from build123d import *

# Parameters (mm, degrees)
SKETCH1_R                = 11.1125
BOSS_EXTRUDE1_DEPTH      = 38.1
BOSS_EXTRUDE2_DEPTH      = 12.7
BOSS_EXTRUDE2_DEPTH_BACK = 12.7
SKETCH2_W                = 9.525
SKETCH2_H                = 31.75
BOSS_EXTRUDE3_DEPTH      = 12.7
BOSS_EXTRUDE3_DEPTH_BACK = 12.7
SKETCH3_W                = 63.5
SKETCH3_H                = 12.7
BOSS_EXTRUDE4_DEPTH      = 12.7
BOSS_EXTRUDE4_DEPTH_BACK = 12.7
SKETCH4_W                = 9.525
SKETCH4_H                = 63.5
BOSS_EXTRUDE5_DEPTH      = 12.7
BOSS_EXTRUDE5_DEPTH_BACK = 12.7


with BuildPart() as part:
    # Sketch1 → Boss-Extrude1 (new body)
    with BuildSketch(Plane(origin=(0, 0, 0), x_dir=(0, 0, -1), z_dir=(1, 0, 0))):
        Circle(SKETCH1_R)
    extrude(amount=-BOSS_EXTRUDE1_DEPTH)

    # Sketch2 → Boss-Extrude2 (add, two sides: drawn at the far end of the back side and taken through both)
    with BuildSketch(Plane.XY.offset(-BOSS_EXTRUDE2_DEPTH_BACK)):
        with Locations((4.7625, 4.7625)):
            Rectangle(SKETCH2_W, SKETCH2_H)
    extrude(amount=BOSS_EXTRUDE2_DEPTH + BOSS_EXTRUDE2_DEPTH_BACK)

    # Sketch3 → Boss-Extrude3 (add, two sides: drawn at the far end of the back side and taken through both)
    with BuildSketch(Plane.XY.offset(-BOSS_EXTRUDE3_DEPTH_BACK)):
        with Locations((-22.225, 26.9875)):
            Rectangle(SKETCH3_W, SKETCH3_H)
    extrude(amount=BOSS_EXTRUDE3_DEPTH + BOSS_EXTRUDE3_DEPTH_BACK)

    # Sketch4 → Boss-Extrude4 (add, two sides: drawn at the far end of the back side and taken through both)
    with BuildSketch(Plane.XY.offset(-BOSS_EXTRUDE4_DEPTH_BACK)):
        with Locations((-49.2125, 52.3875)):
            Rectangle(SKETCH4_W, SKETCH4_H)
    extrude(amount=BOSS_EXTRUDE4_DEPTH + BOSS_EXTRUDE4_DEPTH_BACK)

    # Sketch5 → Boss-Extrude5 (add, two sides: drawn at the far end of the back side and taken through both)
    with BuildSketch(Plane.XY.offset(-BOSS_EXTRUDE5_DEPTH_BACK)):
        Polygon((-53.975, 71.4375), (-41.23944, 71.4375), (-41.23944, 74.6125), (-28.575, 74.6125), (-28.575, 84.1375), (-53.975, 84.1375), align=None)
    extrude(amount=BOSS_EXTRUDE5_DEPTH + BOSS_EXTRUDE5_DEPTH_BACK)


solid = part.part
Design review of the part built by this model. Coordinates are the model's own, in mm. A direction names the side the tool comes from. Coordinates: 2 decimals unless noted, no trailing zeros. Loops run counter-clockwise (first coordinate to the right, second up) from the corner with the lowest first, then second, coordinate; pieces in that order, holes last. Notation, with made-up numbers: M 51,-17.75 L 73,-17.75 A27 cw 73,13.25 Z; hole C 85.5,21 d4. An arc over 180 degrees is marked long. Use one line per item in the form item = value.
(1) Consider section B-B (x = -11). Write out the cut boundary in (y, z) (1 decimal).
Return value:
outline = C 0,0 d22.2; M 20.6,-12.7 L 33.3,-12.7 L 33.3,12.7 L 20.6,12.7 Z
(2) For line 1 along Y through (x, z) = (-32.5, 4); line 2 along Y through (x, z) = (4.5, 2.75); line 3 along Y through (x, z) = (-19.5, 2.25), list the stretches that pass through material, from the lowest coordinate up. Write a range as from..to.
Return value:
line_1 = -10.37..10.37, 20.64..33.34, 74.61..84.14
line_2 = -11.11..33.34
line_3 = -10.88..10.88, 20.64..33.34
(3) Draft analysis for pull direction Y (two halves, no side actions). For faces 1 (the face through (9.525, 11, 0)), 2 (the face through (-41, 84.138, 0)), 3 (the face through (-27, 20.638, 0)), 4 (the face through (5, -11.112, 0)), state which applies: pulls with the +Y half, pulls with the -Y half, needs draft (parallel to the pull), parting line crosses it, or undercut.
Return value:
face_1 = needs draft
face_2 = pulls with the +Y half
face_3 = undercut
face_4 = pulls with the -Y half
(4) Clearance check with flat-ended pins moving along their axes: P1, Ø1.6, axis at y = 73.5, z = 2, coming from the +X side; P2, Ø2.5, axis at x = -42.5, z = -5.5, coming from the -Y side; P3, Ø10, axis at y = 33.5, z = -2.5, coming from the +X side (3 decimals); P4, Ø10, axis at x = -25, y = 1.5, coming from the -Z side. State where each tip first meets the part, or that it passes through.
Return value:
P1 = -41.24
P2 = 20.64
P3 = 9.525
P4 = -11.11
(5) For faces 5 (the face through (-38.1, 0, 0)), 6 (the face through (-28.575, 79, 0)), 7 (the face through (0, 12, 0)), 8 (the face through (-25, 33, -12.7)), 9 (the face through (-18, 33.338, 0)), list the 3-axis set-ups (+Z, -Z, +X, -X, +Y, -Y) from which the entire face can be reached by the end or side of a thin tool; tool diameter is ignored.
Return value:
face_5 = +Z, -Z, -X, -Y
face_6 = +Z, -Z, +X, +Y
face_7 = -X
face_8 = -Z, +X, -X, +Y, -Y
face_9 = +Z, -Z, +X
(6) Consider section C-C (y = 0). Write out the cut boundary in (x, z) (1 decimal), and give its area (3 significant figures).
Return value:
outline = M -38.1,-11.1 L 0,-11.1 L 0,-12.7 L 9.5,-12.7 L 9.5,12.7 L 0,12.7 L 0,11.1 L -38.1,11.1 Z
area = 1,090 mm2
(7) Consider section A-A (x = -35). Write out the cut boundary in (y, z) (1 decimal), and give its area (3 significant figures).
Return value:
outline = C 0,0 d22.2; M 20.6,-12.7 L 33.3,-12.7 L 33.3,12.7 L 20.6,12.7 Z; M 74.6,-12.7 L 84.1,-12.7 L 84.1,12.7 L 74.6,12.7 Z
area = 952 mm2
